Autodesk Inventor part; units mm, degrees
ref_plane "YZ Plane" through (0, 0, 0) normal (1, 0, 0) x (0, 1, 0)
ref_plane "XZ Plane" through (0, 0, 0) normal (0, 1, 0) x (-1, 0, 0)
ref_plane "XY Plane" through (0, 0, 0) normal (0, 0, 1) x (1, 0, 0)
sketch "Sketch1" plane through (0, 0, 0) normal (0, 1, 0) x (-1, 0, 0)
  line L0 (-4, 4) -> (4, 4)
  line L1 (4, 4) -> (4, -4)
  line L2 (4, -4) -> (-4, -4)
  line L3 (-4, -4) -> (-4, 4)
  line L4 (-4, 4) -> (4, -4) construction
  line L5 (4, 4) -> (-4, -4) construction
  circle A0 centre (0, 0) radius 2
  dimension "d0" = 8
  dimension "d1" = 8
  dimension "d2" = 4
extrude "Extrusion1" add sketch "Sketch1" along normal blind 4
thread "Thread1"
properties part number "Ganjal Baut Kutup" material "Copper"
CAD build for the part. Positions are in the model's coordinates, mm. Round coordinates to 2 decimals unless told otherwise and drop trailing zeros. Order: outer loops, then holes, each group sorted by start corner. A loop starts at its lowest first (then second) coordinate and runs counter-clockwise, first axis right, second up. Notation, with made-up numbers: (-5, -3) - (21, -3) arc R19 ccw to (21, 14) - close; hole circle Ø3 at (29, 3). An arc over 180 degrees is marked (long way). Answer as CSV lines item,"result". Start each with the question number.
1. Drill centre lines: L1, parallel to Z at x = 0, y = 2.9; L2, parallel to X at y = 2.9, z = 1.25; L3, parallel to Z at x = 1.75, y = 1. Where is each one in solid material? Low to high. Write a range as [from, to].
2. Saw through at B-B, the plane x = 0. Write the cut outline in (y, z).
3. Pull direction X, two halves, no side cores. Call faces 1 (the face through (-4, 2, 0)), 2 (the face through (4, 2, 0)), 3 (the face through (0, 2, 2)), 4 (the face through (2, 4, 1)): +X half, -X half, draft (parallel to the pull), parting line (faces both ways), or undercut.
4. Saw through at A-A, the plane z = 0. Write the cut outline in (x, y).
Model answer:
1,L1,"z = [-4, -2], [2, 4]"
1,L2,"x = [-4, -1.56], [1.56, 4]"
1,L3,"z = [-4, -0.97], [0.97, 4]"
2,outline,"(0, -4) - (4, -4) - (4, -2) - (0, -2) - close; (0, 2) - (4, 2) - (4, 4) - (0, 4) - close"
3,face 1,"-X half"
3,face 2,"+X half"
3,face 3,"undercut"
3,face 4,"draft"
4,outline,"(-4, 0) - (-2, 0) - (-2, 4) - (-4, 4) - close; (2, 0) - (4, 0) - (4, 4) - (2, 4) - close"
